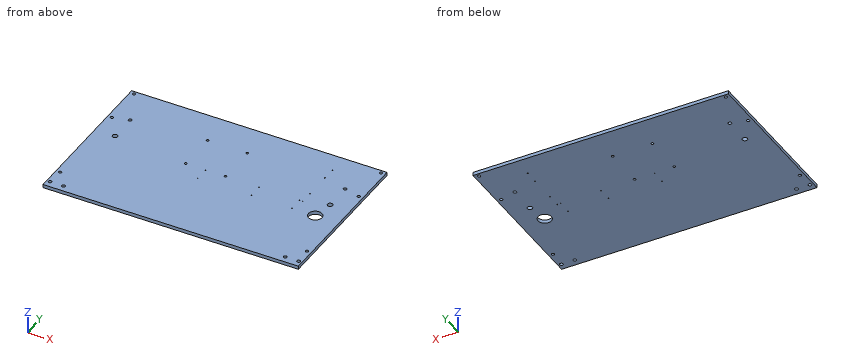
from build123d import *

# Parameters (mm, degrees)
SKETCH1_W           = 482.6
SKETCH1_H           = 304.8
BOSS_EXTRUDE1_DEPTH = 6.35
SKETCH2_R           = 2.7813
CUT_EXTRUDE1_DEPTH  = 286.467638271
SKETCH3_R           = 3.175
CUT_EXTRUDE2_DEPTH  = 286.467638271
SKETCH4_R           = 12.7
CUT_EXTRUDE3_DEPTH  = 286.467638271
SKETCH5_R           = 2.3749
CUT_EXTRUDE4_DEPTH  = 286.467638271
SKETCH6_R           = 3.175
SKETCH6_R_2         = 4.7625
CUT_EXTRUDE5_DEPTH  = 286.467638271
SKETCH7_R           = 0.889
CUT_EXTRUDE6_DEPTH  = 286.467638271
SKETCH8_R           = 0.8255
SKETCH8_R_2         = 0.79375
CUT_EXTRUDE7_DEPTH  = 286.467638271


with BuildPart() as part:
    # Sketch1 → Boss-Extrude1 (new body)
    with BuildSketch(Plane.XY):
        Rectangle(SKETCH1_W, SKETCH1_H)
    extrude(amount=BOSS_EXTRUDE1_DEPTH)

    # Sketch2 → Cut-Extrude1 (cut, through all)
    with BuildSketch(Plane.XY.offset(6.35)):
        with Locations((-233.3498, 146.05)):
            Circle(SKETCH2_R)
        with Locations((-233.3498, -107.95)):
            Circle(SKETCH2_R)
        with Locations((-233.3498, 69.85)):
            Circle(SKETCH2_R)
    cut_extrude1 = extrude(amount=-CUT_EXTRUDE1_DEPTH, mode=Mode.SUBTRACT)

    # Mirror1: Cut-Extrude1 across plane
    add(cut_extrude1.mirror(Plane(origin=(0, 0, 0), x_dir=(0, 0, 1), z_dir=(1, 0, 0))), mode=Mode.SUBTRACT)

    # Sketch3 → Cut-Extrude2 (cut, through all)
    with BuildSketch(Plane.XY.offset(6.35)):
        with Locations((-234.95, -139.7)):
            Circle(SKETCH3_R)
        with Locations((-209.55, -139.7)):
            Circle(SKETCH3_R)
    cut_extrude2 = extrude(amount=-CUT_EXTRUDE2_DEPTH, mode=Mode.SUBTRACT)

    # Mirror2: Cut-Extrude2 across plane
    add(cut_extrude2.mirror(Plane(origin=(0, 0, 0), x_dir=(0, 0, 1), z_dir=(1, 0, 0))), mode=Mode.SUBTRACT)

    # Sketch4 → Cut-Extrude3 (cut, through all)
    with BuildSketch(Plane.XY.offset(6.35)):
        with Locations((196.469, -12.7)):
            Circle(SKETCH4_R)
    extrude(amount=-CUT_EXTRUDE3_DEPTH, mode=Mode.SUBTRACT)

    # Sketch5 → Cut-Extrude4 (cut, through all)
    with BuildSketch(Plane.XY.offset(6.35)):
        with Locations((-62.9, 88.9)):
            Circle(SKETCH5_R)
        with Locations((12.1, 88.9)):
            Circle(SKETCH5_R)
        with Locations((12.1, 13.9)):
            Circle(SKETCH5_R)
        with Locations((-62.9, 13.9)):
            Circle(SKETCH5_R)
    extrude(amount=-CUT_EXTRUDE4_DEPTH, mode=Mode.SUBTRACT)

    # Sketch6 → Cut-Extrude5 (cut, through all)
    with BuildSketch(Plane.XY.offset(6.35)):
        with Locations((-203.2, 77.727111167)):
            Circle(SKETCH6_R)
        with Locations((-203.2, 26.096105915)):
            Circle(SKETCH6_R_2)
        with Locations((203.2, 77.727111167)):
            Circle(SKETCH6_R)
        with Locations((203.2, 26.096105915)):
            Circle(SKETCH6_R_2)
    extrude(amount=-CUT_EXTRUDE5_DEPTH, mode=Mode.SUBTRACT)

    # Sketch7 → Cut-Extrude6 (cut, through all)
    with BuildSketch(Plane.XY.offset(6.35)):
        with Locations((158.821461806, 114.3)):
            Circle(SKETCH7_R)
        with Locations((158.821461806, 88.9)):
            Circle(SKETCH7_R)
        with Locations((158.821461806, 38.1)):
            Circle(SKETCH7_R)
        with Locations((158.821461806, 12.7)):
            Circle(SKETCH7_R)
    extrude(amount=-CUT_EXTRUDE6_DEPTH, mode=Mode.SUBTRACT)

    # Sketch8 → Cut-Extrude7 (cut, through all)
    with BuildSketch(Plane.XY.offset(6.35)):
        with Locations((-25.4, 12.7)):
            Circle(SKETCH8_R)
        with Locations((-25.4, -12.7)):
            Circle(SKETCH8_R)
        with Locations((76.2, 12.7)):
            Circle(SKETCH8_R_2)
        with Locations((76.2, -12.7)):
            Circle(SKETCH8_R_2)
        with Locations((152.4, 12.7)):
            Circle(SKETCH8_R_2)
        with Locations((152.4, -12.7)):
            Circle(SKETCH8_R_2)
    extrude(amount=-CUT_EXTRUDE7_DEPTH, mode=Mode.SUBTRACT)


solid = part.part
Geometry: final body of the model. Coordinates: model frame, mm. Give positions to 0.01 mm unless a question says otherwise; leave off trailing zeros. Write each loop counter-clockwise with the first axis right and the second up, starting at its lowest first coordinate (ties: lowest second). Pieces come first, ordered by that corner, then holes. Notation, with made-up numbers: (-25.5, -29) -> (18.5, -29) arc R20 ccw to (18.5, -6) -> close; hole circle Ø10 at (20.25, -36.5). An arc over 180 degrees is marked (long way). Answer in a Markdown table with one row per item.
(1) Pin query (flat end, axial travel): pin 1 (8.5 mm diameter, centred on x = -203.2, y = 26.1, fed in from +Z). Return the tip coordinate at first contact, or that it passes through.
Answers below:
| item | result |
|---|---|
| pin 1 | through |
(2) Section query A-A on y = -5. Return loops of the section in (x, z).
Answers below:
| item | result |
|---|---|
| outline | (-241.3, 0) -> (186.37, 0) -> (186.37, 6.35) -> (-241.3, 6.35) -> close; (206.57, 0) -> (241.3, 0) -> (241.3, 6.35) -> (206.57, 6.35) -> close |
(3) Ray query, line 1 along Y through (x, z) = (-25.4, 4.25); line 2 along Y through (x, z) = (-62.9, 4); line 3 along X through (y, z) = (70, 3). Return the intervals inside material, ascending. Write a range as [from, to].
Answers below:
| item | result |
|---|---|
| line 1 | [-152.4, -13.53], [-11.87, 11.87], [13.53, 152.4] |
| line 2 | [-152.4, 11.53], [16.27, 86.53], [91.27, 152.4] |
| line 3 | [-241.3, -236.13], [-230.57, 230.57], [236.13, 241.3] |
